Can you work these out from the model? Positions are in its coordinate system, mm. Face numbers are marked on the shaded views. A direction names the side the tool comes from. Round coordinates to 2 decimals unless told otherwise and drop trailing zeros. Write each loop counter-clockwise with the first axis right and the second up, starting at its lowest first coordinate (ties: lowest second). Pieces come first, ordered by that corner, then holes. Notation, with made-up numbers: M 52.25,88 L 110.25,88 A17 ccw 110.25,109 Z; hole C 60.5,87.25 d4. An arc over 180 degrees is marked long. Answer as a JSON object with one key per item and string values. Group by question number.
1) If we mould it in two halves opening along X, with no side actions, what happens to the marked faces 3, 4 and 5? For each: +X half, -X half, draft (parallel to the pull), parting line (faces both ways), or undercut.
2) Suppose I cut it at B-B, the plane y = -3.75. Write out the boundary of the cut face in (x, z), and give its area (3 significant figures).
3) Please list where these lines run through material, in increasing order: L1, parallel to Y at x = 31.25, z = 0.5; L2, parallel to Z at x = 22, y = -25; L3, parallel to X at y = -17, z = 3. Write a range as [from, to].
4) I'm going to push flat-ended pins straight in: pin 1 Ø10 at (y, z) = (-27, 27) entering from +X; pin 2 Ø4 at (x, z) = (17, 12) entering from -Y; pin 3 Ø5 at (x, y) = (31.25, -3.75) entering from +Z; pin 4 Ø3.5 at (x, y) = (3.75, -26.25) entering from -Z. Where does each tip first touch, or does it pass through?
5) Suppose I cut it at D-D, the plane x = 19. Write out the boundary of the cut face in (y, z), and give its area (3 significant figures).
6) On a 3-axis mill with a long thin cutter (end or side, diameter ignored), from which of +Z, -Z, +X, -X, +Y, -Y can I reach the whole of each face in a straight line? I mean the marked faces 1 and 2. Say none if no direction works.
7) Suppose I cut it at C-C, the plane x = 31.25. Write out the boundary of the cut face in (y, z).
8) Suppose I cut it at A-A, the plane x = 23.5. Write out the boundary of the cut face in (y, z).
from build123d import *

# Parameters (mm, degrees)
SKETCH_1_W          = 35
SKETCH_1_H          = 30
EXTRUDE_1_DEPTH     = 1
FILLET_1_R          = 3
SKETCH_2_R          = 2.25
CUT_EXTRUDE_1_DEPTH = 2
SKETCH_3_W          = 1
SKETCH_3_H          = 25
EXTRUDE_2_DEPTH     = 30
CUT_EXTRUDE_2_DEPTH = 27.25
EXTRUDE_3_REACH     = 27.25
SKETCH_5_R          = 2
SKETCH_6_R          = 12.5
EXTRUDE_4_DEPTH     = 7


with BuildPart() as part:
    # ｽｹｯﾁ1 → ﾎﾞｽ - 押し出し1 (new body)
    with BuildSketch(Plane.XY):
        with Locations((17.5, -15)):
            Rectangle(SKETCH_1_W, SKETCH_1_H)
    extrude(amount=EXTRUDE_1_DEPTH)

    # ﾌｨﾚｯﾄ1
    fillet_1_edges = [part.edges().sort_by_distance(p)[0] for p in [
        (0, 0, 0.5),
        (35, 0, 0.5),
        (35, -30, 0.5),
        (0, -30, 0.5),
    ]]
    fillet(fillet_1_edges, radius=FILLET_1_R)

    # ｽｹｯﾁ2 → ｶｯﾄ - 押し出し1 (cut, through all)
    with BuildSketch(Plane.XY.offset(1)):
        with Locations((31.25, -3.75)):
            Circle(SKETCH_2_R)
        with Locations((31.25, -26.25)):
            Circle(SKETCH_2_R)
        with Locations((3.75, -26.25)):
            Circle(SKETCH_2_R)
        with Locations((3.75, -3.75)):
            Circle(SKETCH_2_R)
    extrude(amount=-CUT_EXTRUDE_1_DEPTH, mode=Mode.SUBTRACT)

    # ｽｹｯﾁ3 → ﾎﾞｽ - 押し出し2 (add)
    with BuildSketch(Plane(origin=(0, 0, 0), x_dir=(1, 0, 0), z_dir=(0, 1, 0))):
        with Locations((9.25, -13.5)):
            Rectangle(SKETCH_3_W, SKETCH_3_H)
        with Locations((25.75, -13.5)):
            Rectangle(SKETCH_3_W, SKETCH_3_H)
    extrude(amount=-EXTRUDE_2_DEPTH)

    # ｽｹｯﾁ4 → ｶｯﾄ - 押し出し2 (cut, through all)
    with BuildSketch(Plane(origin=(26.25, 0, 0), x_dir=(0, 0, -1), z_dir=(1, 0, 0))):
        with BuildLine():
            ThreePointArc((-26, -24.5), (-25.757311392, -23.425502313), (-25.076363776, -22.559619304))
            Line((-25.076363776, -22.559619304), (-1, -3))
            Line((-1, -3), (-1, 0))
            Line((-1, 0), (-26, 0))
            Line((-26, 0), (-26, -24.5))
        make_face()
        with BuildLine():
            ThreePointArc((-23.5, -27), (-25.267766953, -26.267766953), (-26, -24.5))
            Line((-26, -24.5), (-26, -30))
            Line((-26, -30), (-1, -30))
            Line((-1, -30), (-1, -27))
            Line((-1, -27), (-23.5, -27))
        make_face()
    extrude(amount=-CUT_EXTRUDE_2_DEPTH, mode=Mode.SUBTRACT)

    # ｽｹｯﾁ5 → ﾎﾞｽ - 押し出し3 (add, up to next)
    with BuildSketch(Plane.ZY.offset(-25.25), mode=Mode.PRIVATE) as extrude_3_sk1:
        with Locations((23.5, -24.5)):
            Circle(SKETCH_5_R)
    extrude_3_tool1 = extrude(extrude_3_sk1.sketch, amount=EXTRUDE_3_REACH, mode=Mode.PRIVATE) - part.part
    add(extrude_3_tool1.solids().sort_by_distance((25.25, -24.5, 23.5))[0])

    # ｽｹｯﾁ6 → ﾎﾞｽ - 押し出し4 (add, symmetric)
    with BuildSketch(Plane(origin=(17.5, 0, 0), x_dir=(0, 0, -1), z_dir=(1, 0, 0))):
        with Locations((-23.5, -24.5)):
            Circle(SKETCH_6_R)
    extrude(amount=EXTRUDE_4_DEPTH, both=True)

    # ｽｹｯﾁ7 → ｶｯﾄ - 回転1 (revolve, cut)
    with BuildSketch(Plane(origin=(0, 0, 23.5), x_dir=(-1, 0, 0), z_dir=(0, 0, -1))):
        Polygon((-24.5, -13), (-19.5, -14.5), (-19.5, -16.5), (-24.5, -22.5), align=None)
        Polygon((-10.5, -13), (-15.5, -14.5), (-15.5, -16.5), (-10.5, -22.5), align=None)
    revolve(axis=Axis((-9.093978877, -24.5, 23.5), (1, 0, 0)), mode=Mode.SUBTRACT)


solid = part.part
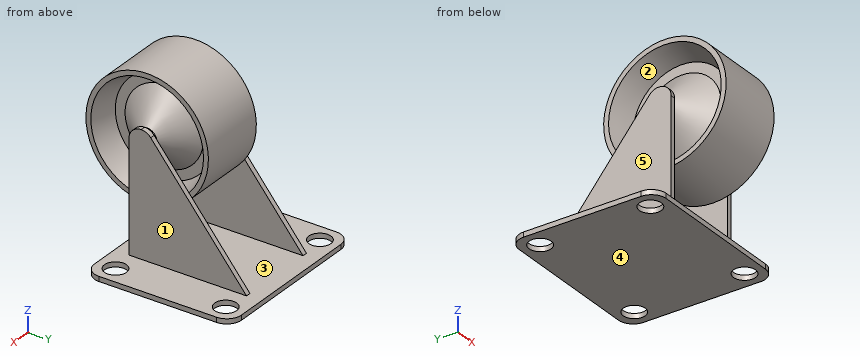
Results:
{
 "1": {"face 3": "undercut", "face 4": "draft", "face 5": "-X half"},
 "2": {"outline": "M 0,0 L 1.5,0 L 1.5,1 L 0,1 Z; M 6,0 L 29,0 L 29,1 L 26.25,1 L 26.25,1.92 L 25.25,1.92 L 25.25,1 L 9.75,1 L 9.75,1.92 L 8.75,1.92 L 8.75,1 L 6,1 Z; M 33.5,0 L 35,0 L 35,1 L 33.5,1 Z", "area": "27.8 mm^2"},
 "3": {"L1": "[-30, -28.5], [-24, -6], [-1.5, 0]", "L2": "[0, 1], [11.01, 12.76], [18.53, 28.47], [34.24, 35.99]", "L3": "[8.75, 9.75], [25.25, 26.25]"},
 "4": {"pin 1": "x = 26.25", "pin 2": "y = -32.62", "pin 3": "z = 1", "pin 4": "through"},
 "5": {"outline": "C -24.5,23.5 d25; M -30,0 L 0,0 L 0,1 L -30,1 Z", "area": "521 mm^2"},
 "6": {"face 1": "+Z, +X, +Y, -Y", "face 2": "none"},
 "7": {"outline": "M -30,0 L -28.5,0 L -28.5,1 L -30,1 Z; M -24,0 L -6,0 L -6,1 L -24,1 Z; M -1.5,0 L 0,0 L 0,1 L -1.5,1 Z"},
 "8": {"outline": "C -24.5,23.5 d25; M -30,0 L 0,0 L 0,1 L -30,1 Z; C -24.5,23.5 d6.4; hole C -24.5,23.5 d22.4"}
}
